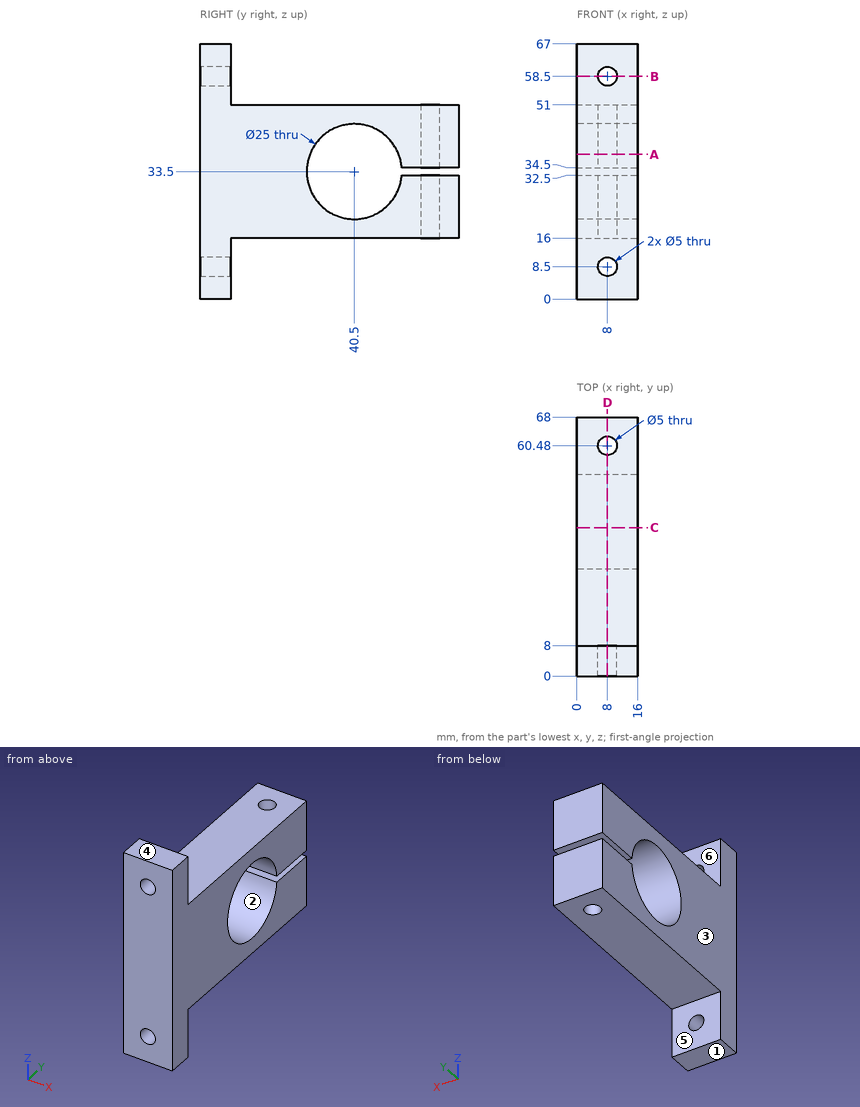
Check sheet for the drawn part. Datum: minimum x, y, z corner. Units: mm. A direction names the side the tool comes from. Coordinates: 2 decimals unless noted, no trailing zeros. Loops run counter-clockwise (first coordinate to the right, second up) from the corner with the lowest first, then second, coordinate; pieces in that order, holes last. Notation, with made-up numbers: (17.5, 53.25) -> (44.5, 53.25) arc R15 cw to (44.5, 65.25) -> close; hole circle Ø5 at (3, 36). An arc over 180 degrees is marked (long way). Answer as a JSON object with one key per item and string values. Group by question number.
Item 1: Depth check by flat-ended pin: pin 1 (6 mm diameter, centred on y = 32.5, z = 32.5, fed in from -X); pin 2 (7.5 mm diameter, centred on x = 7.5, y = 61, fed in from +Z); pin 3 (5 mm diameter, centred on x = 3.5, y = 42, fed in from -Z); pin 4 (5 mm diameter, centred on x = 6.5, z = 7, fed in from +Y). Enter the tip coordinate at first touch or a pass-through.
Item 2: Sectioned sample at C-C on y = 39. Record the boundary of the cut face in (x, z).
Item 3: Sectioned sample at D-D on x = 8. Record the boundary of the cut face in (y, z).
Item 4: Scan lines: probe 1 along Z at (x, y) = (8.5, 41); probe 2 along Z at (x, y) = (11, 63); probe 3 along Y at (x, z) = (9, 37). Record each from-to range of solid material in increasing order.
Item 5: Sectioned sample at B-B on z = 58.5. Record the boundary of the cut face in (x, y), plus the area to 3 significant figures.
Item 6: Sectioned sample at A-A on z = 38. Record the boundary of the cut face in (x, y).
Item 7: Tool access check on the marked faces 4, 5 and 6. Record the directions out of +Z, -Z, +X, -X, +Y, -Y that give a thin tool (end or side, any length) a straight path to the whole face; none if there is none.
Item 8: Mould release check, pull along Z, two halves, no side actions. Record for the marked faces 1, 2 and 3: +Z half, -Z half, draft (parallel to the pull), parting line (faces both ways), or undercut.
Evaluation:
{
 "1": {"pin 1": "passes through", "pin 2": "stops at z = 51", "pin 3": "stops at z = 16", "pin 4": "stops at y = 8"},
 "2": {"outline": "(0, 16) -> (16, 16) -> (16, 21.09) -> (0, 21.09) -> close; (0, 45.91) -> (16, 45.91) -> (16, 51) -> (0, 51) -> close"},
 "3": {"outline": "(0, 0) -> (8, 0) -> (8, 6) -> (0, 6) -> close; (0, 11) -> (8, 11) -> (8, 16) -> (57.98, 16) -> (57.98, 32.5) -> (52.96, 32.5) arc R12.5 cw (long way) to (52.96, 34.5) -> (57.98, 34.5) -> (57.98, 51) -> (8, 51) -> (8, 56) -> (0, 56) -> close; (0, 61) -> (8, 61) -> (8, 67) -> (0, 67) -> close; (62.98, 16) -> (68, 16) -> (68, 32.5) -> (62.98, 32.5) -> close; (62.98, 34.5) -> (68, 34.5) -> (68, 51) -> (62.98, 51) -> close"},
 "4": {"probe 1": "z = 16 to 21.01, 45.99 to 51", "probe 2": "z = 16 to 32.5, 34.5 to 51", "probe 3": "y = 0 to 28.5, 52.5 to 58.19, 62.77 to 68"},
 "5": {"outline": "(0, 0) -> (5.5, 0) -> (5.5, 8) -> (0, 8) -> close; (10.5, 0) -> (16, 0) -> (16, 8) -> (10.5, 8) -> close", "area": "88.0 mm²"},
 "6": {"outline": "(0, 0) -> (16, 0) -> (16, 28.84) -> (0, 28.84) -> close; (0, 52.16) -> (16, 52.16) -> (16, 68) -> (0, 68) -> close; hole circle Ø5 at (8, 60.48)"},
 "7": {"face 4": "+Z, +X, -X, +Y, -Y", "face 5": "-Z, +X, -X, +Y", "face 6": "+Z, +X, -X, +Y"},
 "8": {"face 1": "-Z half", "face 2": "undercut", "face 3": "draft"}
}
